Model file for the job. Use its own axes, mm. Give positions to 0.01 mm unless a question says otherwise; leave off trailing zeros. Loops run counter-clockwise (first coordinate to the right, second up) from the corner with the lowest first, then second, coordinate; pieces in that order, holes last. Notation, with made-up numbers: (4.5, -13) -> (59.5, -13) arc R18 ccw to (59.5, 7) -> close; hole circle Ø4 at (-39, -32). An arc over 180 degrees is marked (long way). Use CSV: the item, a comma, the result in double quotes. Start each with the question number.
(1) Drill centre lines: probe 1 along X at (y, z) = (3.25, -0.2); probe 2 along X at (y, z) = (3.75, -0.05); probe 3 along Y at (x, z) = (287.02, 0.15). Where is each one in solid material? Low to high.
(2) Cut at A-A on y = 5.08. Write the cut outline in (x, z).
(3) Flat gauge pin, fed straight in: pin 1 (3.5 mm diameter, centred on x = 0, y = 5.08, fed in from -Z). Where does the tip first touch, or does it go through?
(4) Cut at B-B on z = -0.1. Write the cut outline in (x, y).
from build123d import *

# Parameters (mm, degrees)
BOSS_EXTRUDE1_DEPTH = 0.5
SKETCH2_R           = 2.032
SKETCH2_R_2         = 2.026725148
CUT_EXTRUDE1_DEPTH  = 2.54


with BuildPart() as part:
    # Sketch1 → Boss-Extrude1 (new, symmetric)
    with BuildSketch(Plane.XY):
        with BuildLine():
            Line((0, 0), (287.02, 0))
            ThreePointArc((287.02, 0), (292.1, 5.08), (287.02, 10.16))
            Line((287.02, 10.16), (0, 10.16))
            ThreePointArc((0, 10.16), (-5.08, 5.08), (0, 0))
        make_face()
    extrude(amount=BOSS_EXTRUDE1_DEPTH, both=True)

    # Sketch2 → Cut-Extrude1 (cut)
    with BuildSketch(Plane.XY.offset(0.5)):
        with Locations((0, 5.08)):
            Circle(SKETCH2_R)
        with Locations((287.02, 5.08)):
            Circle(SKETCH2_R_2)
    extrude(amount=-CUT_EXTRUDE1_DEPTH, mode=Mode.SUBTRACT)


solid = part.part
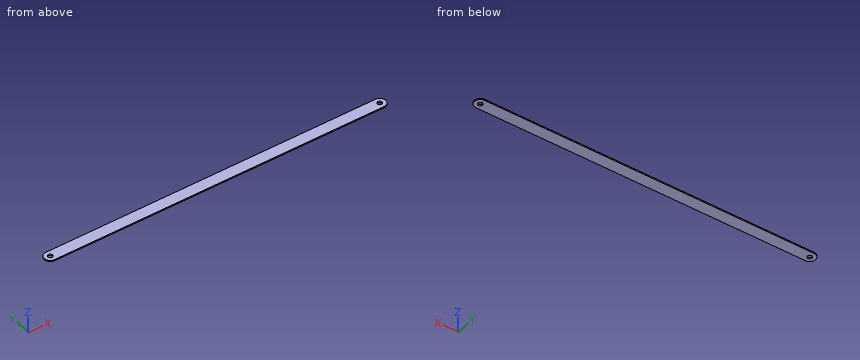
Check result:
1,probe 1,"-4.74 to -0.88, 0.88 to 286.15, 287.89 to 291.76"
1,probe 2,"-4.9 to -1.54, 1.54 to 285.49, 288.55 to 291.92"
1,probe 3,"0 to 3.05, 7.11 to 10.16"
2,outline,"(-5.08, -0.5) -> (-2.03, -0.5) -> (-2.03, 0.5) -> (-5.08, 0.5) -> close; (2.03, -0.5) -> (284.99, -0.5) -> (284.99, 0.5) -> (2.03, 0.5) -> close; (289.05, -0.5) -> (292.1, -0.5) -> (292.1, 0.5) -> (289.05, 0.5) -> close"
3,pin 1,"through"
4,outline,"(0, 0) -> (287.02, 0) arc R5.08 ccw to (287.02, 10.16) -> (0, 10.16) arc R5.08 ccw to start; hole circle Ø4.06 at (0, 5.08); hole circle Ø4.05 at (287.02, 5.08)"
